Source: CAD feature listing. Evaluate the final solid. Frame: model axes, mm. Face numbers are marked on the shaded views. A direction names the side the tool comes from. Give positions to 0.01 mm unless a question says otherwise; leave off trailing zeros. Order: outer loops, then holes, each group sorted by start corner. A loop starts at its lowest first (then second) coordinate and runs counter-clockwise, first axis right, second up.
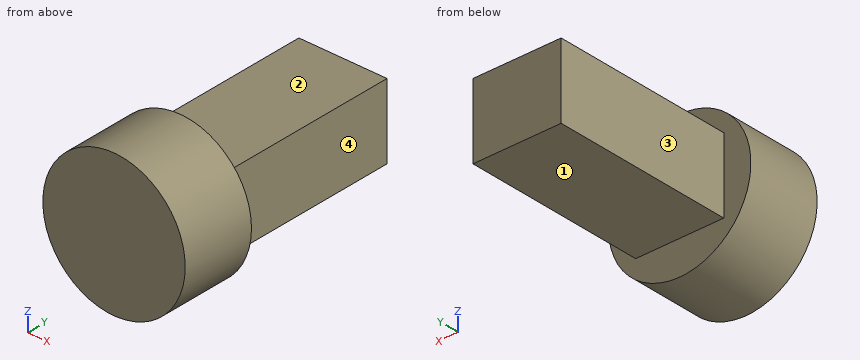
Solid Edge part; units mm, degrees
sketch "Sketch1" plane through (0, 0, 0) normal (0, 0, 1) x (1, 0, 0)
  line L0 (6.5, -13.5) -> (-6.5, -13.5)
  line L1 (-6.5, -13.5) -> (-6.5, 13.5)
  line L2 (-6.5, 13.5) -> (6.5, 13.5)
  line L3 (6.5, 13.5) -> (6.5, -13.5)
  dimension "D1" = 6.5
  dimension "D2" = 6.5
extrude "Protrusion1" add sketch "Sketch1" against normal blind 11
sketch "Sketch2" plane through (0, -13.5, -5.5) normal (0, -1, 0) x (1, 0, 0)
  circle A0 centre (0, 0) radius 10.5
extrude "Extrusionsausprägung_2" add sketch "Sketch2" along normal blind 11
1) Section query D-D on y = 4. Output: boundary loops of the cut face in (x, z), and give its area (3 significant figures).
Checks:
outline: (-6.5, -11) - (6.5, -11) - (6.5, 0) - (-6.5, 0) - close
area: 143 mm2
2) Section query B-B on x = 5.5. Output: boundary loops of the cut face in (y, z), and give its area (3 significant figures).
Checks:
outline: (-24.5, -14.44) - (-13.5, -14.44) - (-13.5, -11) - (13.5, -11) - (13.5, 0) - (-13.5, 0) - (-13.5, 3.44) - (-24.5, 3.44) - close
area: 494 mm2
3) Section query C-C on y = -21. Output: boundary loops of the cut face in (x, z), and give its area (3 significant figures).
Checks:
outline: circle Ø21 at (0, -5.5)
area: 346 mm2
4) Reachability of the marked faces 1, 2, 3 and 4 from +Z, -Z, +X, -X, +Y, -Y: full face, straight path, thin tool, end or side. Return the list, or none.
Checks:
face 1: -Z, +X, -X, +Y
face 2: +Z, +X, -X, +Y
face 3: +Z, -Z, -X, +Y
face 4: +Z, -Z, +X, +Y
5) First-contact query: pin 1 Ø5 at (y, z) = (-12.5, -0.5) entering from +X; pin 2 Ø10 at (y, z) = (8.5, 2.5) entering from +X; pin 3 Ø12 at (y, z) = (-15.5, -13.5) entering from -X. Flat tips, straight axial feed; report the tip coordinate or a pass-through.
Checks:
pin 1: stops at x = 10.14
pin 2: stops at x = 6.5
pin 3: stops at x = -10.31
6) Ray query, L1, parallel to Z at x = -1, y = 3; L2, parallel to X at y = -11.5, z = -3; L3, parallel to Y at x = 5, z = -13.5. Return the intervals inside material, ascending.
Checks:
L1: z = -11 to 0
L2: x = -6.5 to 6.5
L3: y = -24.5 to -13.5
7) Section query A-A on z = -5.5. Output: boundary loops of the cut face in (x, y), and give its area (3 significant figures).
Checks:
outline: (-10.5, -24.5) - (10.5, -24.5) - (10.5, -13.5) - (6.5, -13.5) - (6.5, 13.5) - (-6.5, 13.5) - (-6.5, -13.5) - (-10.5, -13.5) - close
area: 582 mm2
